from build123d import *

# Parameters (mm, degrees)
F0_W = 304.8
F0_H = 25.4
F2_T = -2.54


# Not quite as in the source:
# - a fillet or chamfer that OpenCascade refuses, or shapes differently, is made with other operations: its cross-section is extruded or revolved along the edge and cut away or added


with BuildPart() as f1:
    # F0 (on Right) → F1 (revolve)
    with BuildSketch(Plane.YZ):
        Rectangle(F0_W, F0_H)
    revolve(axis=Axis((0, 0, -12.7), (0, -1, 0)))

    # F2
    f2_openings = [f1.faces().sort_by_distance(p)[0] for p in [
        (0, 152.4, -12.7),
        (0, -152.4, -12.7),
    ]]
    offset(amount=F2_T, openings=f2_openings)

    # F3: fillet of radius 22.86 on 1 edges, made by hand

    # F3_s1 → F3_t2 (revolve, cut)
    with BuildSketch(Plane.YZ):
        with BuildLine():
            ThreePointArc((141.9273117109, 12.7), (147.3154653836, 12.0559267194), (152.4, 10.16))
            Line((152.4, 10.16), (152.4, 12.7))
            Line((152.4, 12.7), (141.9273117109, 12.7))
        make_face()
    revolve(axis=Axis((0, 152.4, -12.7), (0, -1, 0)), mode=Mode.SUBTRACT)


solid = f1.part
Geometry: final body of the model. Coordinates: model frame, mm. Give positions to 0.01 mm unless a question says otherwise; leave off trailing zeros. Order: outer loops, then holes, each group sorted by start corner. A loop starts at its lowest first (then second) coordinate and runs counter-clockwise, first axis right, second up. Notation, with made-up numbers: (10, -3) - (18, -3) arc R28 cw to (18, 29) - close; hole circle Ø2 at (69.25, 84). An arc over 180 degrees is marked (long way). Use CSV: the item, a comma, the result in double quotes.
1. Section query A-A (y = 78.5). Output: boundary loops of the cut face in (x, z), plus the area to 3 significant figures.
Answers below:
outline,"circle Ø50.8 at (0, -12.7); hole circle Ø45.72 at (0, -12.7)"
area,"385 mm2"
2. Material intervals for line 1 along Z through (x, y) = (0, -91); line 2 along X through (y, z) = (-112, -12); line 3 along X through (y, z) = (-53, -12.7), sorted ascending. Write a range as from..to.
Answers below:
line 1,"-38.1..-35.56, 10.16..12.7"
line 2,"-25.39..-22.85, 22.85..25.39"
line 3,"-25.4..-22.86, 22.86..25.4"
3. Mould query, pull axis X, two halves, no side actions, for faces 1 (the face through (-4, -152.4, 10)), 2 (the face through (-7.629, -3.176, 11.527)), 3 (the face through (-15.45, 2.13, -29.55)). Classes: +X half, -X half, draft (parallel to the pull), parting line (faces both ways), or undercut.
Answers below:
face 1,"draft"
face 2,"parting line"
face 3,"undercut"
4. Contact query for flat-ended pins moving along their axis: pin 1 (8 mm diameter, centred on y = 23, z = -29.5, fed in from +X); pin 2 (10 mm diameter, centred on x = 14, y = -34.5, fed in from -Z); pin 3 (5 mm diameter, centred on y = -50, z = 5.5, fed in from +X). Output: stop coordinate, or through.
Answers below:
pin 1,"x = 21.94"
pin 2,"z = -36.45"
pin 3,"x = 19.97"
